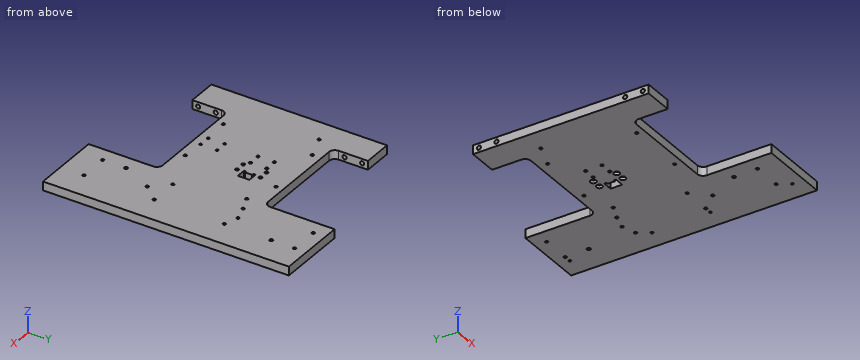
```python
from build123d import *

# Parameters (mm, degrees)
SKETCH_1_W                     = 391
SKETCH_1_H                     = 180
EXTRUDE_1_DEPTH                = 15
SKETCH_3_W                     = 9.5
SKETCH_3_H                     = 15.8
CUT_EXTRUDE_2_DEPTH            = 431.704074743
SKETCH_4_W                     = 13.5
SKETCH_4_H                     = 19.8
CUT_EXTRUDE_3_DEPTH            = 431.704074743
SKETCH_6_W                     = 100
SKETCH_6_H                     = 15
EXTRUDE_2_DEPTH                = 120
SKETCH_7_W                     = 100
SKETCH_7_H                     = 15
EXTRUDE_3_DEPTH                = 120
FILLET_1_R                     = 10
SKETCH_8_W                     = 41
SKETCH_8_H                     = 180
CUT_EXTRUDE_5_DEPTH            = 120
FILLET_2_R                     = 10
SKETCH_9_W                     = 50
SKETCH_9_H                     = 15
EXTRUDE_4_DEPTH                = 60
SKETCH_10_W                    = 50
SKETCH_10_H                    = 15
EXTRUDE_5_DEPTH                = 60
SKETCH_11_W                    = 20
SKETCH_11_H                    = 120
EXTRUDE_6_DEPTH                = 15
FILLET_3_R                     = 10
SKETCH_12_W                    = 3
SKETCH_12_H                    = 3.9
CUT_EXTRUDE_6_DEPTH            = 462.221205063
SKETCH_13_R                    = 3.5
CUT_EXTRUDE_7_DEPTH            = 425.529150943
HOLE_WIZARD_M5_1_D             = 4.2
HOLE_WIZARD_M5_1_DEPTH         = 12.4
HOLE_WIZARD_M5_1_TIP           = 1.2618073
HOLE_WIZARD_M6_1_D             = 5
HOLE_WIZARD_M6_1_DEPTH         = 15
HOLE_WIZARD_M6_1_TIP           = 1.502151548
HOLE_WIZARD_M6_2_D             = 5
HOLE_WIZARD_M6_2_DEPTH         = 15
HOLE_WIZARD_M6_2_TIP           = 1.502151548
HOLE_WIZARD_M5_1_2_D           = 5.8
HOLE_WIZARD_M5_1_2_CBORE_D     = 10
HOLE_WIZARD_M5_1_2_CBORE_DEPTH = 5
HOLE_WIZARD_M6_3_D             = 5
HOLE_WIZARD_M6_3_DEPTH         = 15
HOLE_WIZARD_M6_3_TIP           = 1.502151548
HOLE_WIZARD_M6_4_D             = 5
HOLE_WIZARD_M6_4_DEPTH         = 15
HOLE_WIZARD_M6_4_TIP           = 1.502151548
HOLE_WIZARD_M5_2_D             = 4.2
HOLE_WIZARD_M5_2_DEPTH         = 12.4
HOLE_WIZARD_M5_2_TIP           = 1.2618073
SKETCH_28_R                    = 3
CUT_EXTRUDE_8_DEPTH            = 462.221205063


with BuildPart() as part:
    # 草图1 → 凸台-拉伸1 (new body)
    with BuildSketch(Plane.XY):
        with Locations((195.5, 90)):
            Rectangle(SKETCH_1_W, SKETCH_1_H)
    extrude(amount=EXTRUDE_1_DEPTH)

    # 草图3 → 切除-拉伸2 (cut, through all)
    with BuildSketch(Plane.XY.offset(15)):
        with Locations((178.45, 115.45)):
            Rectangle(SKETCH_3_W, SKETCH_3_H)
    extrude(amount=-CUT_EXTRUDE_2_DEPTH, mode=Mode.SUBTRACT)

    # 草图4 → 切除-拉伸3 (cut, through all)
    with BuildSketch(Plane.XY.offset(15)):
        with Locations((178.45, 115.45)):
            Rectangle(SKETCH_4_W, SKETCH_4_H)
    extrude(amount=-CUT_EXTRUDE_3_DEPTH, mode=Mode.SUBTRACT)

    # 草图6 → 凸台-拉伸2 (add)
    with BuildSketch(Plane(origin=(0, 180, 0), x_dir=(1, 0, 0), z_dir=(0, 1, 0))):
        with Locations((280, -7.5)):
            Rectangle(SKETCH_6_W, SKETCH_6_H)
    extrude(amount=EXTRUDE_2_DEPTH)

    # 草图7 → 凸台-拉伸3 (add)
    with BuildSketch(Plane.XZ):
        with Locations((280, 7.5)):
            Rectangle(SKETCH_7_W, SKETCH_7_H)
    extrude(amount=EXTRUDE_3_DEPTH)

    # 圆角1
    fillet_1_edges = [part.edges().sort_by_distance(p)[0] for p in [
        (230, 0, 7.5),
        (230, 180, 7.5),
    ]]
    fillet(fillet_1_edges, radius=FILLET_1_R)

    # 草图8 → 切除-拉伸5 (cut)
    with BuildSketch(Plane.XY.offset(15)):
        with Locations((370.5, 90)):
            Rectangle(SKETCH_8_W, SKETCH_8_H)
    extrude(amount=-CUT_EXTRUDE_5_DEPTH, mode=Mode.SUBTRACT)

    # 圆角2
    fillet_2_edges = [part.edges().sort_by_distance(p)[0] for p in [
        (330, 0, 7.5),
        (330, 180, 7.5),
    ]]
    fillet(fillet_2_edges, radius=FILLET_2_R)

    # 草图9 → 凸台-拉伸4 (add)
    with BuildSketch(Plane(origin=(0, 180, 0), x_dir=(1, 0, 0), z_dir=(0, 1, 0))):
        with Locations((25, -7.5)):
            Rectangle(SKETCH_9_W, SKETCH_9_H)
    extrude(amount=EXTRUDE_4_DEPTH)

    # 草图10 → 凸台-拉伸5 (add)
    with BuildSketch(Plane.XZ):
        with Locations((25, 7.5)):
            Rectangle(SKETCH_10_W, SKETCH_10_H)
    extrude(amount=EXTRUDE_5_DEPTH)

    # 草图11 → 凸台-拉伸6 (add)
    with BuildSketch(Plane.XY.offset(15)):
        with Locations((340, -60)):
            Rectangle(SKETCH_11_W, SKETCH_11_H)
        with Locations((340, 240)):
            Rectangle(SKETCH_11_W, SKETCH_11_H)
    extrude(amount=-EXTRUDE_6_DEPTH)

    # 圆角3
    fillet_3_edges = [part.edges().sort_by_distance(p)[0] for p in [
        (50, 0, 7.5),
        (50, 180, 7.5),
    ]]
    fillet(fillet_3_edges, radius=FILLET_3_R)

    # 草图12 → 切除-拉伸6 (cut, through all)
    with BuildSketch(Plane(origin=(0, 0, 0), x_dir=(-1, 0, 0), z_dir=(0, 0, -1))):
        with Locations((-170.2, 107.5)):
            Rectangle(SKETCH_12_W, SKETCH_12_H)
        with Locations((-170.2, 123.4)):
            Rectangle(SKETCH_12_W, SKETCH_12_H)
    extrude(amount=-CUT_EXTRUDE_6_DEPTH, mode=Mode.SUBTRACT)

    # 草图13 → 切除-拉伸7 (cut, through all)
    with BuildSketch(Plane(origin=(50, 0, 0), x_dir=(0, 0, -1), z_dir=(1, 0, 0))):
        with Locations((-7.5, -50)):
            Circle(SKETCH_13_R)
        with Locations((-7.5, -20)):
            Circle(SKETCH_13_R)
        with Locations((-7.5, 230)):
            Circle(SKETCH_13_R)
        with Locations((-7.5, 200)):
            Circle(SKETCH_13_R)
    extrude(amount=-CUT_EXTRUDE_7_DEPTH, mode=Mode.SUBTRACT)

    # Hole Wizard M5 _1
    with Locations(Plane(origin=(0, 0, 0), x_dir=(-1, 0, 0), z_dir=(0, 0, -1))):
        with Locations((-316, 280), (-316.471513322, 140), (-316, 40), (-316, -100)):
            Hole(HOLE_WIZARD_M5_1_D / 2, depth=HOLE_WIZARD_M5_1_DEPTH)
            with Locations((0, 0, -(HOLE_WIZARD_M5_1_DEPTH + HOLE_WIZARD_M5_1_TIP / 2))):  # 118° drill point
                Cone(0, HOLE_WIZARD_M5_1_D / 2, HOLE_WIZARD_M5_1_TIP, mode=Mode.SUBTRACT)

    # M6 螺纹孔1
    with Locations(Plane(origin=(0, 0, 0), x_dir=(-1, 0, 0), z_dir=(0, 0, -1))):
        with Locations((-280, 167.5), (-180, 167.5), (-80, 164.6), (-280, 12.5), (-180, 12.5), (-80, 12.5)):
            Hole(HOLE_WIZARD_M6_1_D / 2, depth=HOLE_WIZARD_M6_1_DEPTH)
            with Locations((0, 0, -(HOLE_WIZARD_M6_1_DEPTH + HOLE_WIZARD_M6_1_TIP / 2))):  # 118° drill point
                Cone(0, HOLE_WIZARD_M6_1_D / 2, HOLE_WIZARD_M6_1_TIP, mode=Mode.SUBTRACT)

    # M6 螺纹孔2
    with Locations(Plane(origin=(0, 0, 0), x_dir=(-1, 0, 0), z_dir=(0, 0, -1))):
        with Locations((-125.8, 129.45), (-145.8, 129.45), (-145.8, 101.45), (-125.8, 101.45)):
            Hole(HOLE_WIZARD_M6_2_D / 2, depth=HOLE_WIZARD_M6_2_DEPTH)
            with Locations((0, 0, -(HOLE_WIZARD_M6_2_DEPTH + HOLE_WIZARD_M6_2_TIP / 2))):  # 118° drill point
                Cone(0, HOLE_WIZARD_M6_2_D / 2, HOLE_WIZARD_M6_2_TIP, mode=Mode.SUBTRACT)

    # Hole Wizard M5 _1 2 (through all)
    with Locations(Plane(origin=(0, 0, 0), x_dir=(-1, 0, 0), z_dir=(0, 0, -1))):
        with Locations((-171.3, 95.45), (-155.3, 95.45), (-171.3, 135.45), (-155.3, 135.45)):
            CounterBoreHole(HOLE_WIZARD_M5_1_2_D / 2, HOLE_WIZARD_M5_1_2_CBORE_D / 2, HOLE_WIZARD_M5_1_2_CBORE_DEPTH)

    # M6 螺纹孔3
    with Locations(Plane.XY.offset(15)):
        with Locations((304, 280), (255, 280), (255, 160), (304, 160), (304, -80), (255, -80), (255, 40), (304, 40)):
            Hole(HOLE_WIZARD_M6_3_D / 2, depth=HOLE_WIZARD_M6_3_DEPTH)
            with Locations((0, 0, -(HOLE_WIZARD_M6_3_DEPTH + HOLE_WIZARD_M6_3_TIP / 2))):  # 118° drill point
                Cone(0, HOLE_WIZARD_M6_3_D / 2, HOLE_WIZARD_M6_3_TIP, mode=Mode.SUBTRACT)

    # M6 螺纹孔4
    with Locations(Plane(origin=(0, 0, 0), x_dir=(-1, 0, 0), z_dir=(0, 0, -1))):
        with Locations((-40, 150), (-230, 150)):
            Hole(HOLE_WIZARD_M6_4_D / 2, depth=HOLE_WIZARD_M6_4_DEPTH)
            with Locations((0, 0, -(HOLE_WIZARD_M6_4_DEPTH + HOLE_WIZARD_M6_4_TIP / 2))):  # 118° drill point
                Cone(0, HOLE_WIZARD_M6_4_D / 2, HOLE_WIZARD_M6_4_TIP, mode=Mode.SUBTRACT)

    # M5 螺纹孔2
    with Locations(Plane.XY.offset(15)):
        with Locations((123.5, 43), (143.5, 43), (143.5, 15), (123.5, 15)):
            Hole(HOLE_WIZARD_M5_2_D / 2, depth=HOLE_WIZARD_M5_2_DEPTH)
            with Locations((0, 0, -(HOLE_WIZARD_M5_2_DEPTH + HOLE_WIZARD_M5_2_TIP / 2))):  # 118° drill point
                Cone(0, HOLE_WIZARD_M5_2_D / 2, HOLE_WIZARD_M5_2_TIP, mode=Mode.SUBTRACT)

    # 草图28 → 切除-拉伸8 (cut, through all)
    with BuildSketch(Plane.XY.offset(15)):
        with Locations((304, 240)):
            Circle(SKETCH_28_R)
        with Locations((255, -40)):
            Circle(SKETCH_28_R)
    extrude(amount=-CUT_EXTRUDE_8_DEPTH, mode=Mode.SUBTRACT)


solid = part.part
```
The listing builds one solid part. Answer for the finished solid, in the listing's coordinates (mm). Coordinates: 2 decimals unless noted, no trailing zeros. Write each loop counter-clockwise with the first axis right and the second up, starting at its lowest first coordinate (ties: lowest second). Pieces come first, ordered by that corner, then holes. Notation, with made-up numbers: M -15.5,-18 L 21.5,-18 A33 ccw 21.5,20 Z; hole C 6.5,12 d11. An arc over 180 degrees is marked long. Use a Markdown table: item, result. Add a question column.
1. Section B-B (x = 191) is taken. Give the vertices of the cut face in (y, z), plus the area to 3 significant figures.
2. Given P1, Ø8, axis at x = 255, y = -80, coming from the +Z side; P2, Ø4, axis at x = 108.5, z = 10.5, coming from the +Y side; P3, Ø3, axis at x = 80, y = 164.6, coming from the -Z side; P4, Ø9.5, axis at x = 155.3, y = 95.45, coming from the -Z side, each flat-ended and moving along its own axis, determine where each tip first touches the part or whether it passes through.
3. Straight lines are drawn through the part: line 1 along X through (y, z) = (150.5, 1.75); line 2 along X through (y, z) = (238.5, 9.5); line 3 along Y through (x, z) = (304, 7.5). For each, find the intervals that lie inside material, in ascending order. Write a range as [from, to].
4. Section A-A (z = 7.75) is taken. Count the separate pieces of the cut face and the enclosed holes in it, plus the area to 3 significant figures.
Data:
| question | item | result |
|---|---|---|
| 1 | outline | M 0,0 L 180,0 L 180,15 L 0,15 Z |
| 1 | area | 2,700 mm2 |
| 2 | P1 | stops at z = 15 |
| 2 | P2 | stops at y = 180 |
| 2 | P3 | passes through |
| 2 | P4 | stops at z = 5 |
| 3 | line 1 | x = [0, 37.55], [42.45, 227.55], [232.45, 350] |
| 3 | line 2 | x = [0, 50], [230, 301.4], [306.6, 350] |
| 3 | line 3 | y = [-120, -82.5], [-77.5, 37.5], [42.5, 157.5], [162.5, 237], [243, 277.5], [282.5, 300] |
| 4 | separate pieces | 5 |
| 4 | enclosed holes | 35 |
| 4 | area | 95,500 mm2 |
